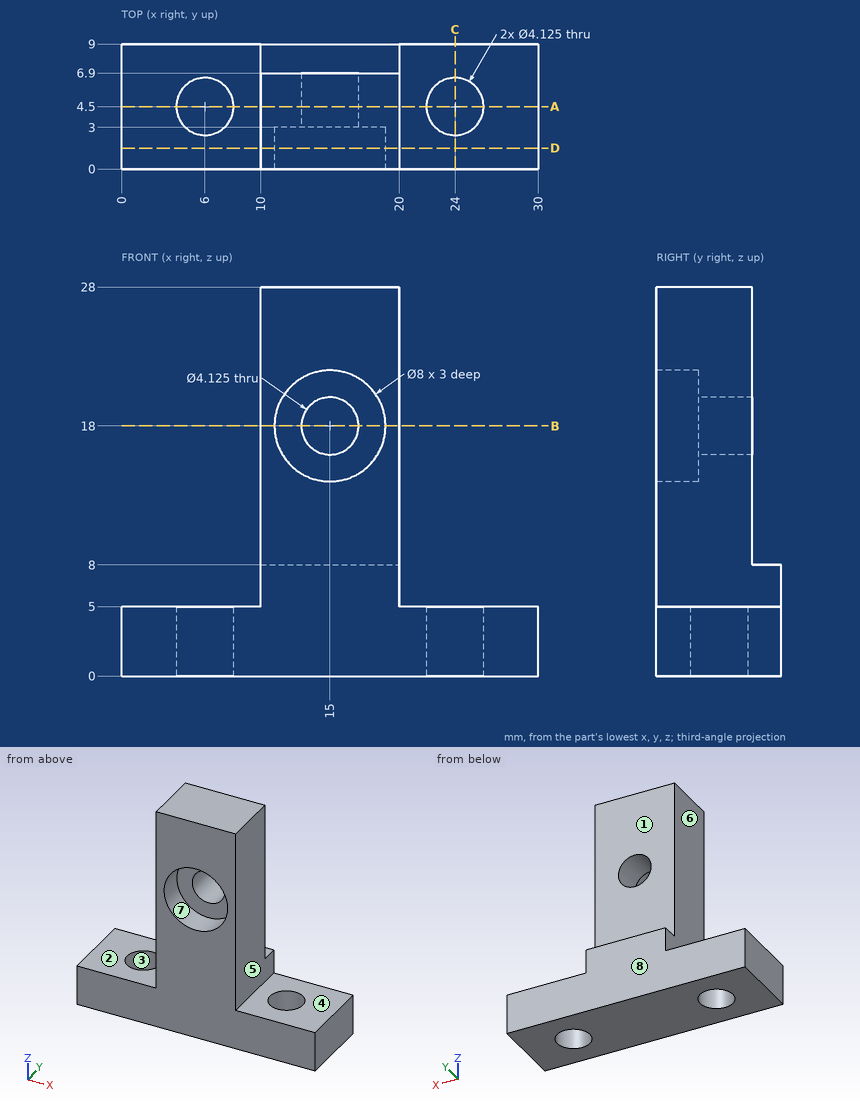
Input: dimensioned drawing with shaded views. Units: mm. Origin: part minimum x, y, z. A direction names the side the tool comes from. Give positions to 0.01 mm unless a question says otherwise; leave off trailing zeros. Loops run counter-clockwise (first coordinate to the right, second up) from the corner with the lowest first, then second, coordinate; pieces in that order, holes last. Notation, with made-up numbers: (49, 32.5) -> (82, 32.5) arc R21 ccw to (82, 45.5) -> close; hole circle Ø11 at (83.25, 22.25). An arc over 180 degrees is marked (long way). Use a Markdown table: item, result. Add a question column.
1) Reachability of the marked faces 1, 2, 3 and 4 from +Z, -Z, +X, -X, +Y, -Y: full face, straight path, thin tool, end or side. Return the list, or none.
2) Section query C-C, the plane x = 24. Return the cut outline in (y, z).
3) Pull-direction query (X, two-part tool) for the marked faces 5, 6, 7 and 8; classes: +X half, -X half, draft (parallel to the pull), parting line (faces both ways), or undercut.
4) Section query B-B, the plane z = 18. Return the cut outline in (x, y).
5) Section query A-A, the plane y = 4.5. Return the cut outline in (x, z) (1 decimal), then the cut area to 3 significant figures.
6) Section query D-D, the plane y = 1.5. Return the cut outline in (x, z), then the cut area to 3 significant figures.
7) First-contact query: pin 1 (2.5 mm diameter, centred on y = 4.5, z = 12, fed in from -X); pin 2 (6.5 mm diameter, centred on x = 15, z = 18, fed in from -Y); pin 3 (3 mm diameter, centred on x = 15, z = 17, fed in from +Y); pin 4 (1.5 mm diameter, centred on y = 8, z = 20, fed in from +X). Flat tips, straight axial feed; report the tip coordinate or a pass-through.
8) Line query: line 1 along Y through (x, z) = (6, 2.9); line 2 along X through (y, z) = (6, 2.5); line 3 along Z through (x, y) = (15, 2.35). Output: solid intervals per line, ascending. Write a range as [from, to].
Numbers:
| question | item | result |
|---|---|---|
| 1 | face 1 | +Z, +X, -X, +Y |
| 1 | face 2 | +Z, -X, +Y, -Y |
| 1 | face 3 | +Z, -Z |
| 1 | face 4 | +Z, +X, +Y, -Y |
| 2 | outline | (0, 0) -> (2.44, 0) -> (2.44, 5) -> (0, 5) -> close; (6.56, 0) -> (9, 0) -> (9, 5) -> (6.56, 5) -> close |
| 3 | face 5 | +X half |
| 3 | face 6 | -X half |
| 3 | face 7 | undercut |
| 3 | face 8 | draft |
| 4 | outline | (10, 0) -> (11, 0) -> (11, 3) -> (12.94, 3) -> (12.94, 6.9) -> (10, 6.9) -> close; (17.06, 3) -> (19, 3) -> (19, 0) -> (20, 0) -> (20, 6.9) -> (17.06, 6.9) -> close |
| 5 | outline | (0, 0) -> (3.9, 0) -> (3.9, 5) -> (0, 5) -> close; (8.1, 0) -> (21.9, 0) -> (21.9, 5) -> (20, 5) -> (20, 28) -> (10, 28) -> (10, 5) -> (8.1, 5) -> close; (26.1, 0) -> (30, 0) -> (30, 5) -> (26.1, 5) -> close; hole circle Ø4.1 at (15, 18) |
| 5 | area | 325 mm2 |
| 6 | outline | (0, 0) -> (30, 0) -> (30, 5) -> (20, 5) -> (20, 28) -> (10, 28) -> (10, 5) -> (0, 5) -> close; hole circle Ø8 at (15, 18) |
| 6 | area | 330 mm2 |
| 7 | pin 1 | stops at x = 10 |
| 7 | pin 2 | stops at y = 3 |
| 7 | pin 3 | stops at y = 6.9 |
| 7 | pin 4 | passes through |
| 8 | line 1 | y = [0, 2.44], [6.56, 9] |
| 8 | line 2 | x = [0, 4.58], [7.42, 22.58], [25.42, 30] |
| 8 | line 3 | z = [0, 14], [22, 28] |
